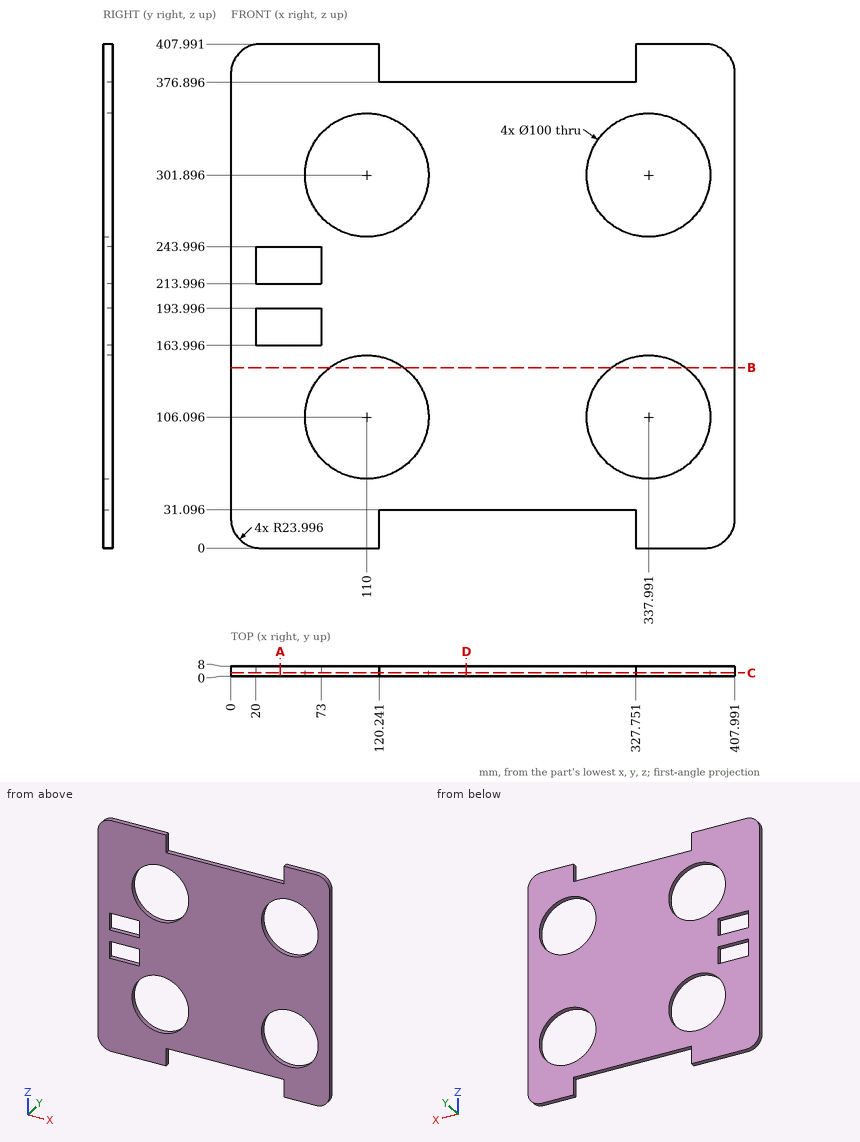
The figure shows three views and two pictorial views of one solid part (mm, origin at its lowest corner). Answer the questions. Round coordinates to 2 decimals unless told otherwise and drop trailing zeros. Write each loop counter-clockwise with the first axis right and the second up, starting at its lowest first coordinate (ties: lowest second). Pieces come first, ordered by that corner, then holes. Notation, with made-up numbers: (-7.75, 60) - (6.25, 60) arc R16 cw to (6.25, 77) - close; hole circle Ø6 at (32, 76.25). An arc over 180 degrees is marked (long way). Use one line per item in the form item = value. Start each with the question number.
Item 1: Flat-ended cylindrical pins translate along their axes: pin 1 Ø2 at (x, y) = (183, 3) entering from +Z; pin 2 Ø1.5 at (x, y) = (213, 7) entering from -Z; pin 3 Ø4 at (y, z) = (5, 14) entering from -X. Find the tip coordinate at first contact, or state that the pin passes through.
Item 2: A cutting plane is placed at A-A (x = 40). Write down the section's boundary in (y, z) (1 decimal), plus the area to 3 significant figures.
Item 3: A cutting plane is placed at D-D (x = 190.5). Write down the section's boundary in (y, z) (1 decimal).
Item 4: A cutting plane is placed at C-C (y = 2.5). Give the number of separate pieces and of enclosed holes in the cut face, plus the area to 3 significant figures.
Item 5: Find the intervals of material crossed by line 1 (Z direction, x = 339.5, y = 7); line 2 (X direction, y = 2.25, z = 324.5); line 3 (X direction, y = 2.75, z = 136.5) (1 decimal), in increasing order. Write a range as [from, to].
Item 6: A cutting plane is placed at B-B (z = 146). Write down the section's boundary in (x, y) (1 decimal).
The answers:
q1.pin_1 = 376.9
q1.pin_2 = 31.1
q1.pin_3 = 1.37
q2.outline = (0, 0) - (8, 0) - (8, 164) - (0, 164) - close; (0, 194) - (8, 194) - (8, 214) - (0, 214) - close; (0, 244) - (8, 244) - (8, 408) - (0, 408) - close
q2.area = 2,780 mm^2
q3.outline = (0, 31.1) - (8, 31.1) - (8, 376.9) - (0, 376.9) - close
q4.separate_pieces = 1
q4.enclosed_holes = 6
q4.area = 118,000 mm^2
q5.line_1 = [0, 56.12], [156.07, 251.92], [351.87, 407.99]
q5.line_2 = [0, 65.4], [154.6, 293.39], [382.59, 407.99]
q5.line_3 = [0, 70.3], [149.7, 298.3], [377.7, 408]
q6.outline = (0, 0) - (79.9, 0) - (79.9, 8) - (0, 8) - close; (140.1, 0) - (307.9, 0) - (307.9, 8) - (140.1, 8) - close; (368.1, 0) - (408, 0) - (408, 8) - (368.1, 8) - close
